Part model, mm, in its own coordinate system. Coordinates: 2 decimals unless noted, no trailing zeros. Use a Markdown table: item, result. Add a question column.
Q1. Wall check: L1, parallel to Y at x = -90, z = -1.75; L2, parallel to X at y = -20, z = -0.5; L3, parallel to Y at x = -68, z = 0.5. Give the ranges that are in metal, low to high. Write a range as from..to.
Q2. Slice it at A-A on z = -2.5. Count the separate pieces of the cut face and the enclosed holes in it, then the cut area to 3 significant figures.
Q3. Pin check, flat tips, straight feed: pin 1 Ø10.5 at (x, y) = (61.82, 72.13) entering from +Z; pin 2 Ø3 at (y, z) = (29.5, 3) entering from -X; pin 3 Ø1 at (y, z) = (49.5, 3) entering from +X; pin 4 Ø2 at (y, z) = (-59.5, 1.5) entering from +X. Stop position of each tip, or through.
from build123d import *

# Parameters (mm, degrees)
SKETCH5_R               = 125
SKETCH5_R_2             = 32
BOSS_EXTRUDE2_DEPTH     = 4
CUT_EXTRUDE1_REACH      = 178.958
SKETCH7_R               = 4.5
CIRPATTERN1_COUNT       = 5
FILL_START              = -4
FILL_PATTERN1_OUTLINE_R = 4.5
FILL_PATTERN1_DEPTH     = 8
FILLET1_R               = 6.5


# Read off the part's stored shape, not the designer's step: Fill Pattern1
with BuildPart() as part:
    # Sketch5 → Boss-Extrude2 (new, symmetric)
    with BuildSketch(Plane.XY):
        Circle(SKETCH5_R)
        Circle(SKETCH5_R_2, mode=Mode.SUBTRACT)
    extrude(amount=BOSS_EXTRUDE2_DEPTH, both=True)

    # Sketch7 → Cut-Extrude1 (cut, up to next)
    with BuildSketch(Plane.XY.offset(4), mode=Mode.PRIVATE) as cut_extrude1_sk1:
        with BuildLine():
            ThreePointArc((-9.355894551, 30.601752191), (0, 32), (9.355894551, 30.601752191))
            Line((9.355894551, 30.601752191), (19.588904216, 64.07241865))
            ThreePointArc((19.588904216, 64.07241865), (0, 67), (-19.588904216, 64.07241865))
            Line((-19.588904216, 64.07241865), (-9.355894551, 30.601752191))
        make_face()
    cut_extrude1_tool1 = extrude(cut_extrude1_sk1.sketch, amount=-CUT_EXTRUDE1_REACH, mode=Mode.PRIVATE) & part.part
    # Sketch7 → Cut-Extrude1 (cut, up to next)
    with BuildSketch(Plane.XY.offset(4), mode=Mode.PRIVATE) as cut_extrude1_sk2:
        with Locations((-26.450336353, 36.405764747)):
            Circle(SKETCH7_R)
    cut_extrude1_tool2 = extrude(cut_extrude1_sk2.sketch, amount=-CUT_EXTRUDE1_REACH, mode=Mode.PRIVATE) & part.part
    cut_extrude1_1 = cut_extrude1_tool1.solids().sort_by_distance((0, 50.80907, 4))[0]
    add(cut_extrude1_1, mode=Mode.SUBTRACT)
    cut_extrude1_2 = cut_extrude1_tool2.solids().sort_by_distance((-26.450336, 36.405765, 4))[0]
    add(cut_extrude1_2, mode=Mode.SUBTRACT)
    cut_extrude1 = cut_extrude1_1 + cut_extrude1_2  # Cut-Extrude1 as one shape, for the pattern or mirror that repeats it

    # CirPattern1: Cut-Extrude1 ×5 about axis
    cirpattern1_axis = Axis((0, 0, 0), (0, 0, 1))
    for i in range(1, CIRPATTERN1_COUNT):
        add(cut_extrude1.rotate(cirpattern1_axis, i * 360 / CIRPATTERN1_COUNT), mode=Mode.SUBTRACT)

    # Fill Pattern1 outline → Fill Pattern1 (cut)
    with BuildSketch(Plane.XY.offset(FILL_START)):
        with Locations((-94.985534108, 1.657978305)):
            Circle(FILL_PATTERN1_OUTLINE_R)
        with Locations((-92.413711498, -22.016051139)):
            Circle(FILL_PATTERN1_OUTLINE_R)
        with Locations((-84.035195714, -44.306731139)):
            Circle(FILL_PATTERN1_OUTLINE_R)
        with Locations((-70.376439715, -63.813456292)):
            Circle(FILL_PATTERN1_OUTLINE_R)
        with Locations((-52.295673376, -79.310547317)):
            Circle(FILL_PATTERN1_OUTLINE_R)
        with Locations((-30.928977742, -89.824264989)):
            Circle(FILL_PATTERN1_OUTLINE_R)
        with Locations((-7.618900879, -94.69399376)):
            Circle(FILL_PATTERN1_OUTLINE_R)
        with Locations((16.169899353, -93.613750663)):
            Circle(FILL_PATTERN1_OUTLINE_R)
        with Locations((38.942685147, -86.651411343)):
            Circle(FILL_PATTERN1_OUTLINE_R)
        with Locations((59.268558619, -74.244445187)):
            Circle(FILL_PATTERN1_OUTLINE_R)
        with Locations((75.870370386, -57.172427506)):
            Circle(FILL_PATTERN1_OUTLINE_R)
        with Locations((87.704967558, -36.508055959)):
            Circle(FILL_PATTERN1_OUTLINE_R)
        with Locations((94.028738868, -13.549749009)):
            Circle(FILL_PATTERN1_OUTLINE_R)
        with Locations((94.444338509, 10.259938485)):
            Circle(FILL_PATTERN1_OUTLINE_R)
        with Locations((88.925652827, 33.424956292)):
            Circle(FILL_PATTERN1_OUTLINE_R)
        with Locations((77.819441139, 54.489761147)):
            Circle(FILL_PATTERN1_OUTLINE_R)
        with Locations((61.823547572, 72.13077389)):
            Circle(FILL_PATTERN1_OUTLINE_R)
        with Locations((41.943052947, 85.239544812)):
            Circle(FILL_PATTERN1_OUTLINE_R)
        with Locations((19.427121857, 92.992401626)):
            Circle(FILL_PATTERN1_OUTLINE_R)
        with Locations((-4.30948694, 94.902203823)):
            Circle(FILL_PATTERN1_OUTLINE_R)
        with Locations((-27.775315017, 90.84895151)):
            Circle(FILL_PATTERN1_OUTLINE_R)
        with Locations((-49.495918093, 81.087325434)):
            Circle(FILL_PATTERN1_OUTLINE_R)
        with Locations((-68.106510795, 66.230684464)):
            Circle(FILL_PATTERN1_OUTLINE_R)
        with Locations((-82.437721138, 47.212525991)):
            Circle(FILL_PATTERN1_OUTLINE_R)
        with Locations((-91.58906647, 25.227830854)):
            Circle(FILL_PATTERN1_OUTLINE_R)
    extrude(amount=FILL_PATTERN1_DEPTH, mode=Mode.SUBTRACT)

    # Fillet1
    fillet1_edges = [part.edges().sort_by_distance(p)[0] for p in [
        (19.588904216, 64.07241865, 0),
        (9.355894551, 30.601752191, 0),
        (-9.355894551, 30.601752191, 0),
        (-19.588904216, 64.07241865, 0),
        (-53.508579173, -40.321606551, 0),
        (-25.556336322, -19.258080741, 0),
        (-10.418180943, -30.256594419, 0),
        (-21.813066349, -63.349744565, 0),
        (21.813066349, -63.349744565, 0),
        (10.418180943, -30.256594419, 0),
        (25.556336322, -19.258080741, 0),
        (53.508579173, -40.321606551, 0),
        (66.989795575, 1.169311231, 0),
        (31.995126245, 0.558477006, 0),
        (26.212865417, 18.354445963, 0),
        (54.883186967, 38.429621236, 0),
        (-54.883186967, 38.429621236, 0),
        (-31.995126245, 0.558477006, 0),
        (-66.989795575, 1.169311231, 0),
    ]]
    fillet(fillet1_edges, radius=FILLET1_R)


solid = part.part
Recorded:
| question | item | result |
|---|---|---|
| 1 | L1 | -86.75..-25.81, -18.22..21.02, 29.44..86.75 |
| 1 | L2 | -123.39..-96.44, -88.39..-28.16, 28.16..123.39 |
| 1 | L3 | -104.89..-67.63, -59.99..61.73, 70.73..104.89 |
| 2 | separate pieces | 1 |
| 2 | enclosed holes | 31 |
| 2 | area | 38,900 mm² |
| 3 | pin 1 | z = 4 |
| 3 | pin 2 | x = -121.82 |
| 3 | pin 3 | x = 115 |
| 3 | pin 4 | x = 110.47 |
